Design review of the part built by this model. Coordinates are the model's own, in mm. A direction names the side the tool comes from. Coordinates: 2 decimals unless noted, no trailing zeros. Write each loop counter-clockwise with the first axis right and the second up, starting at its lowest first coordinate (ties: lowest second). Pieces come first, ordered by that corner, then holes. Notation, with made-up numbers: (-33.75, -6) - (-4.75, -6) arc R15 ccw to (-4.75, 23) - close; hole circle Ø1 at (38, 23.25). An arc over 180 degrees is marked (long way). One line per item, written item: value.
from build123d import *

# Parameters (mm, degrees)
EXTRUDE_THIN1_DEPTH = 7.62


with BuildPart() as part:
    # Sketch1 → Extrude-Thin1 (new body)
    with BuildSketch(Plane.XY):
        Polygon((0, 0), (-2.54, 0), (-3.175, 0.846666667), (-3.175, 1.905), (-2.032, 1.905), (-2.032, 3.175), (-4.445, 3.175), (-4.445, 0.423333333), (-3.175, -1.27), (0, -1.27), align=None)
    extrude(amount=EXTRUDE_THIN1_DEPTH)

    # Mirror1: part across plane


with BuildPart() as part_1:
    add(part.part)
    add(part.part.mirror(Plane(origin=(0, 0, 7.62), x_dir=(0, 0, 1), z_dir=(1, 0, 0))))


solid = part_1.part
1. Mouldability with a two-part tool opening along X and no side actions: class faces 4 (the face through (-3, 3.175, 4)), 5 (the face through (3.175, 1, 4)), 6 (the face through (2.853, 0.417, 3.757)), 7 (the face through (3.82, -0.41, 3.76)) as released by +X, released by -X, zero draft, split by the parting line, or undercut.
Answer block:
face 4: zero draft
face 5: undercut
face 6: undercut
face 7: released by +X
2. Consider section D-D, the plane x = 1.25. Write out the cut boundary in (y, z), then the cut area to 3 significant figures.
Answer block:
outline: (-1.27, 0) - (0, 0) - (0, 7.62) - (-1.27, 7.62) - close
area: 9.68 mm^2
3. Insertion check: pin 1 Ø1 at (y, z) = (0, 6) entering from -X (3 decimals). The pin has a flat end and moves straight along its axis. Give the tip position at first contact, or say it passes through.
Answer block:
pin 1: stops at x = -4.445
4. Consider section C-C, the plane z = 4.5. Write out the cut boundary in (x, y) (3 decimals).
Answer block:
outline: (-4.445, 0.423) - (-3.175, -1.27) - (3.175, -1.27) - (4.445, 0.423) - (4.445, 3.175) - (2.032, 3.175) - (2.032, 1.905) - (3.175, 1.905) - (3.175, 0.847) - (2.54, 0) - (-2.54, 0) - (-3.175, 0.847) - (-3.175, 1.905) - (-2.032, 1.905) - (-2.032, 3.175) - (-4.445, 3.175) - close
5. Consider section B-B, the plane x = -3. Write out the cut boundary in (y, z) (3 decimals).
Answer block:
outline: (-1.27, 0) - (0.613, 0) - (0.613, 7.62) - (-1.27, 7.62) - close; (1.905, 0) - (3.175, 0) - (3.175, 7.62) - (1.905, 7.62) - close
6. Consider section A-A, the plane y = 1.65. Write out the cut boundary in (x, z) (3 decimals).
Answer block:
outline: (-4.445, 0) - (-3.175, 0) - (-3.175, 7.62) - (-4.445, 7.62) - close; (3.175, 0) - (4.445, 0) - (4.445, 7.62) - (3.175, 7.62) - close
7. For faces 1 (the face through (-2.853, 0.417, 3.757)), 2 (the face through (0.1, -0.5, 7.62)), 3 (the face through (2.032, 3, 4)), list the 3-axis set-ups (+Z, -Z, +X, -X, +Y, -Y) from which the entire face can be reached by the end or side of a thin tool; tool diameter is ignored.
Answer block:
face 1: +Z, -Z
face 2: +Z, +X, -X, +Y, -Y
face 3: +Z, -Z, +Y
8. Wall thickness on line 1 along X through (y, z) = (2.15, 6.25) (3 decimals); line 2 along X through (y, z) = (1, 2.25) (3 decimals); line 3 along Y through (x, z) = (2.25, 1.5) (3 decimals): over which ranges is each line inside the solid? List them lowest first.
Answer block:
line 1: x = -4.445 to -2.032, 2.032 to 4.445
line 2: x = -4.445 to -3.175, 3.175 to 4.445
line 3: y = -1.27 to 0, 1.905 to 3.175
